Here's how the part is built. I have some questions about the finished solid (model axes, mm). Round coordinates to 2 decimals unless told otherwise and drop trailing zeros. Write each loop counter-clockwise with the first axis right and the second up, starting at its lowest first coordinate (ties: lowest second). Pieces come first, ordered by that corner, then holes. Notation, with made-up numbers: (80.5, 63.25) -> (137.5, 63.25) arc R6 ccw to (137.5, 74.25) -> close; hole circle Ø4 at (52.25, 5.5). An arc over 180 degrees is marked (long way). Answer as CSV lines item,"result".
```python
from build123d import *

# Parameters (mm, degrees)
F0_W     = 44.034278
F0_H     = 38.278166
F0_R     = 7.855569
F1_DEPTH = 44.45
F2_R     = 5.08
F3_R     = 5.08


with BuildPart() as f1:
    # F0 (on Top) → F1 (new body)
    with BuildSketch(Plane.XY):
        with Locations((0.719513, 0.431709)):
            Rectangle(F0_W, F0_H)
        Circle(F0_R, mode=Mode.SUBTRACT)
    extrude(amount=F1_DEPTH)

    # F2
    f2_edges = [f1.edges().sort_by_distance(p)[0] for p in [
        (0.719513, -18.707374, 44.45),
        (22.736652, 0.431709, 44.45),
        (0.719513, 19.570792, 44.45),
        (-21.297626, 0.431709, 44.45),
    ]]
    fillet(f2_edges, radius=F2_R)

    # F3
    f3_edges = [f1.edges().sort_by_distance(p)[0] for p in [
        (0.719513, 19.570792, 0),
        (-21.297626, 0.431709, 0),
        (0.719513, -18.707374, 0),
        (22.736652, 0.431709, 0),
    ]]
    fillet(f3_edges, radius=F3_R)


solid = f1.part
```
1. Suppose I cut it at B-B on y = 0. Please give me the cut outline in (x, z), and give its area (3 significant figures).
Numbers:
outline,"(-21.3, 5.08) arc R5.08 ccw to (-16.22, 0) -> (-7.86, 0) -> (-7.86, 44.45) -> (-16.22, 44.45) arc R5.08 ccw to (-21.3, 39.37) -> close; (7.86, 0) -> (17.66, 0) arc R5.08 ccw to (22.74, 5.08) -> (22.74, 39.37) arc R5.08 ccw to (17.66, 44.45) -> (7.86, 44.45) -> close"
area,"1,240 mm^2"
2. Suppose I cut it at A-A on x = 0. Please give me the cut outline in (y, z), and give its area (3 significant figures).
Numbers:
outline,"(-18.71, 5.08) arc R5.08 ccw to (-13.63, 0) -> (-7.86, 0) -> (-7.86, 44.45) -> (-13.63, 44.45) arc R5.08 ccw to (-18.71, 39.37) -> close; (7.86, 0) -> (14.49, 0) arc R5.08 ccw to (19.57, 5.08) -> (19.57, 39.37) arc R5.08 ccw to (14.49, 44.45) -> (7.86, 44.45) -> close"
area,"981 mm^2"
3. If we mould it in two halves opening along X, with no side actions, what happens to faces 1 (the face through (4, 7, 0)), 2 (the face through (7.493, 2.36, 21.914)), 3 (the face through (21.29, 0.7, 42.92)), 4 (the face through (-19.85, 0.7, 1.53))? For each: released by +X, released by -X, zero draft, split by the parting line, or undercut.
Numbers:
face 1,"zero draft"
face 2,"undercut"
face 3,"released by +X"
face 4,"released by -X"
4. Suppose I cut it at C-C on z = 26. Please give me the cut outline in (x, y).
Numbers:
outline,"(-21.3, -18.71) -> (22.74, -18.71) -> (22.74, 19.57) -> (-21.3, 19.57) -> close; hole circle Ø15.71 at (0, 0)"
5. If I drill on line 1 (Y direction, x = 0, z = 21); line 2 (Y direction, x = 6, z = 4.5); line 3 (Z direction, x = 0.5, y = 15), over which ranges is the centre line in solid material (lowest first)?
Numbers:
line 1,"y = -18.71 to -7.86, 7.86 to 19.57"
line 2,"y = -18.67 to -5.07, 5.07 to 19.54"
line 3,"z = 0.03 to 44.42"
6. Suppose I cut it at D-D on z = 3.5. Please give me the cut outline in (x, y).
Numbers:
outline,"(-21.05, -18.46) -> (22.48, -18.46) -> (22.48, 19.32) -> (-21.05, 19.32) -> close; hole circle Ø15.71 at (0, 0)"
